Part model, mm, in its own coordinate system. Face numbers are marked on the shaded views. A direction names the side the tool comes from. Give positions to 0.01 mm unless a question says otherwise; leave off trailing zeros. Order: outer loops, then holes, each group sorted by start corner. A loop starts at its lowest first (then second) coordinate and runs counter-clockwise, first axis right, second up. Notation, with made-up numbers: (70, 8) - (101, 8) arc R20 ccw to (101, 31) - close; hole circle Ø7 at (-33, 25.25). An arc over 180 degrees is marked (long way). One line per item, written item: value.
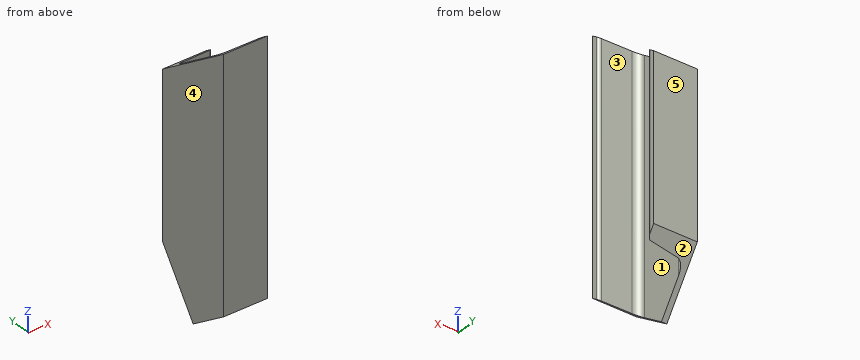
Autodesk Inventor part; units mm, degrees
ref_plane "Начальная плоскость" through (0, 0, 0) normal (0, 0, 1) x (1, 0, 0)
ref_plane "Конечная плоскость" through (0, 0, 226.4162) normal (0, 0, 1) x (1, 0, 0)
ref_plane "РабПлоскость8" through (-29, -423.958, 290.4468) normal (0, -0.5651746, -0.8249713) x (1, 0, 0)
ref_plane "Начальная плоскость" through (0, 0, 0) normal (0, 0, 1) x (1, 0, 0)
ref_plane "Конечная плоскость" through (0, 0, 226.4162) normal (0, 0, 1) x (1, 0, 0)
sketch "Эскиз" plane through (0, 0, 0) normal (0, 0, 1) x (1, 0, 0)
  line L0 (36, -32.5) -> (0, -32.5)
  line L1 (36, -32.5) -> (36, -28.696)
  line L2 (33.6994, -26.2039) -> (9.9215, -24.3017)
  line L3 (4.4, -18.3208) -> (4.4, 18.3208)
  line L4 (33.6994, 26.2039) -> (9.9215, 24.3017)
  line L5 (36, 28.696) -> (36, 32.5)
  line L6 (0, 32.5) -> (36, 32.5)
  line L7 (0, -32.5) -> (0, 32.5)
  arc A0 (4.4, -18.3208) -> (9.9215, -24.3017) centre (10.4, -18.3208) ccw
  arc A1 (9.9215, 24.3017) -> (4.4, 18.3208) centre (10.4, 18.3208) ccw
  arc A2 (36, -28.696) -> (33.6994, -26.2039) centre (33.5, -28.696) ccw
  arc A3 (33.6994, 26.2039) -> (36, 28.696) centre (33.5, 28.696) ccw
  line L8 (0, 45.5) -> (0, -45.5) construction
  line L9 (-7.2974, 0) -> (43.7847, 0) construction
  point P0 (36, -26.388)
  point P1 (4.4, -23.86)
  point P2 (4.4, 23.86)
  point P3 (36, 26.388)
  dimension "d3" = 36
  dimension "d5" = 4.4
  dimension "d7" = 65
  dimension "d9" = 8.64
  dimension "d11" = 8.64
  dimension "d13" = 6.112
  dimension "d15" = 6.112
  dimension "d22" = 6
  dimension "d23" = 2.5
  dimension "d24" = 32.5
  dimension "d25" = 0
extrude "Тело" add sketch "Эскиз" along normal up to surface (226.4162 mm away) from surface at 0
sketch "Sketch3" plane through (0, 0, 0) normal (0, 0, 1) x (1, 0, 0)
  line L0 (0, 0) -> (10, 0)
ref_plane "Work Plane7" through (0, 0, 0) normal (0, -1, 0) x (1, 0, 0)
sketch "Sketch4" plane through (0, 0, 0) normal (0, -1, 0) x (1, 0, 0)
  line L0 (-2, 0) -> (12, 0)
  line L1 (-2, 226.4162) -> (12, 226.4162)
  dimension "d29" = 226.4162
ref_plane "РабПлоскость8" through (-29, -423.958, 290.4468) normal (0, -0.5651746, -0.8249713) x (1, 0, 0)
split "Разделение1" plane through (-29, -423.958, 290.4468) removes the side toward (0, -0.5651746, -0.8249713)
ref_plane "РабПлоскость9" through (36, -560.5141, 590.2499) normal (0, 0.5674011, 0.8234416) x (1, 0, 0)
split "Разделение2" plane through (36, -560.5141, 590.2499) removes the side toward (0, 0.5674011, 0.8234416)
ref_plane "РабПлоскость10" through (36, 95.3234, 138.3382) normal (0, 0.8234416, -0.5674011) x (1, 0, 0)
split "Разделение3" plane through (36, 95.3234, 138.3382) removes the side toward (0, 0.8234416, -0.5674011)
equation "\"d3\" = b"
equation "\"d7\" = ParH"
equation "\"d22\" = R"
equation "\"d23\" = R1"
equation "\"d24\" = 0.5 * d7"
equation "\"d16\" = G_L"
equation "\"R1\" = 2.5"
equation "\"R\" = 6"
equation "\"t1\" = 4.4"
equation "\"t2\" = 7.2"
equation "\"ParH\" = 65"
equation "\"b\" = 36"
equation "\"msp_x1\" = 0.04 * b"
equation "\"msp_x2\" = -0.08 * t1 + 0.04 * b"
equation "\"G_L\" = d29"
equation "\"ex\" = 0"
equation "\"G_OFFSET_START\" = 0"
equation "\"G_OFFSET_END\" = 22.18382"
equation "\"d27\" = G_OFFSET_END + B_L"
equation "\"B_L\" = 204.2324"
properties part number "Швеллер 6.5U-226,42 ГОСТ 8240-97" material "Сталь, мягкая"
1) Two-plate mould, pull along Y, no slides. Class the marked faces 3, 4 and 5: pulls with the +Y half, pulls with the -Y half, needs draft (parallel to the pull), parting line crosses it, or undercut.
Answer:
face 3: undercut
face 4: needs draft
face 5: pulls with the +Y half
2) Slice it at B-B on z = 55. Write the cut outline in (x, y).
Answer:
outline: (0, -32.5) - (36, -32.5) - (36, -28.7) arc R2.5 ccw to (33.7, -26.2) - (9.92, -24.3) arc R6 cw to (4.4, -18.32) - (4.4, 18.32) arc R6 cw to (9.92, 24.3) - (33.7, 26.2) arc R2.5 ccw to (36, 28.7) - (36, 32.5) - (0, 32.5) - close
3) Slice it at C-C on x = 13.5. Write the cut outline in (y, z), then the cut area to 3 significant figures.
Answer:
outline: (-32.5, 22.27) - (-24.59, 16.84) - (-24.59, 220.96) - (-32.5, 226.42) - close; (24.59, 35.68) - (32.5, 47.17) - (32.5, 181.63) - (24.59, 187.08) - close
area: 2,750 mm2
4) Wall check: line 1 along Y through (x, z) = (10, 180.5); line 2 along X through (y, z) = (-0.5, 54); line 3 along Y through (x, z) = (19.5, 143). Give the ranges that are in metal, low to high. Write a range as [from, to].
Answer:
line 1: y = [-32.5, -24.31], [24.31, 32.5]
line 2: x = [0, 4.4]
line 3: y = [-32.5, -25.07], [25.07, 32.5]
5) Slice it at A-A on x = 28. Write the cut outline in (y, z).
Answer:
outline: (-32.5, 22.27) - (-25.75, 17.64) - (-25.75, 221.76) - (-32.5, 226.42) - close; (25.75, 37.37) - (32.5, 47.17) - (32.5, 181.63) - (25.75, 186.28) - close
6) Drop flat-ended pins along their axis: P1, Ø11, axis at y = 4, z = 139.5, coming from the +X side; P2, Ø12, axis at y = -22, z = 28, coming from the +X side; P3, Ø10, axis at x = 11, z = 39, coming from the +Y side. Give the stop position or say it passes through.
Answer:
P1: stops at x = 4.4
P2: stops at x = 35.9
P3: stops at y = 30.32
7) Slice it at D-D on z = 196.5. Write the cut outline in (x, y), then the cut area to 3 significant figures.
Answer:
outline: (0, -32.5) - (36, -32.5) - (36, -28.7) arc R2.5 ccw to (33.7, -26.2) - (9.92, -24.3) arc R6 cw to (4.4, -18.32) - (4.4, 10.92) - (0, 10.92) - close
area: 429 mm2
8) Which spindle directions (+Z, -Z, +X, -X, +Y, -Y) get a long thin tool onto all of the face, cutting with end or side? Do the marked faces 1 and 2. Say none if no direction does.
Answer:
face 1: +Z, -Z, +X
face 2: -Z, +X, -X, +Y
